```python
from build123d import *

# Parameters (mm, degrees)
SKETCH_R        = 1.6
PAD_DEPTH       = 9.5
SKETCH001_R     = 1.6
POCKET_DEPTH    = 8.001
POCKET_FACE6_W  = 8
POCKET_FACE6_H  = 9.5
PAD001_DEPTH    = 10
SKETCH002_R     = 1.6
POCKET001_DEPTH = 8.001


with BuildPart() as part:
    # Sketch → Pad (new body)
    with BuildSketch(Plane.XY):
        with BuildLine():
            ThreePointArc((0, -4), (4, 0), (0, 4))
            Line((0, 4), (-20, 4))
            Line((-20, 4), (-20, -4))
            Line((-20, -4), (0, -4))
        make_face()
        Circle(SKETCH_R, mode=Mode.SUBTRACT)
    extrude(amount=PAD_DEPTH)

    # Sketch001 (on Face2 of Pad) → Pocket (cut, through all)
    with BuildSketch(Plane(origin=(0, 4, 0), x_dir=(-1, 0, 0), z_dir=(0, 1, 0))):
        with Locations((15, 4.75)):
            Circle(SKETCH001_R)
    extrude(amount=-POCKET_DEPTH, mode=Mode.SUBTRACT)

    # Pocket Face6 → Pad001 (add)
    with BuildSketch(Plane(origin=(-20, 0, 4.75), x_dir=(0, 1, 0), z_dir=(-1, 0, 0))):
        Rectangle(POCKET_FACE6_W, POCKET_FACE6_H)
    extrude(amount=PAD001_DEPTH)

    # Sketch002 (on Face8 of Pad001) → Pocket001 (cut, through all)
    with BuildSketch(Plane(origin=(0, 4, 0), x_dir=(-1, 0, 0), z_dir=(0, 1, 0))):
        with Locations((25, 4.75)):
            Circle(SKETCH002_R)
    extrude(amount=-POCKET001_DEPTH, mode=Mode.SUBTRACT)


solid = part.part
```
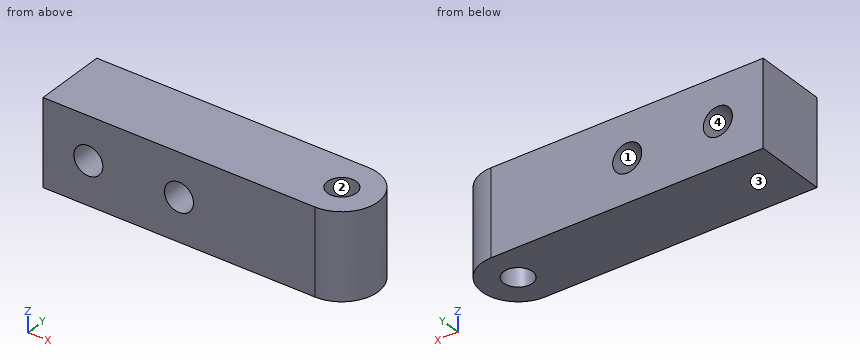
The listing builds one solid part. Answer for the finished solid, in the listing's coordinates (mm). Face numbers are marked on the shaded views. Coordinates: 2 decimals unless noted, no trailing zeros. Loops run counter-clockwise (first coordinate to the right, second up) from the corner with the lowest first, then second, coordinate; pieces in that order, holes last. Notation, with made-up numbers: (34.25, -40) - (85.25, -40) arc R11 ccw to (85.25, -23) - close; hole circle Ø6 at (88.25, 54). An arc over 180 degrees is marked (long way). Use a Markdown table: item, result. Add a question column.
1) The part is cut by section C-C, the plane x = -15. Give the vertices of the cut face in (y, z), and give its area (3 significant figures).
2) The part is cut by section B-B, the plane y = 0. Give the vertices of the cut face in (x, z), and give its area (3 significant figures).
3) The part is cut by section A-A, the plane z = 4.75. Give the vertices of the cut face in (x, y), and give its area (3 significant figures).
4) The part is cut by section D-D, the plane z = 1.75. Give the vertices of the cut face in (x, y), and give its area (3 significant figures).
5) Find the intervals of material crossed by line 1 (Z direction, x = -15, y = 0.75); line 2 (Y direction, x = -0.5, z = 7); line 3 (X direction, y = -1.25, z = 1), in increasing order.
6) The mould has two halves that part along Z. Classify the marked faces 1, 2, 3 and 4: released by +Z, released by -Z, zero draft, split by the parting line, or undercut.
Here are the results:
| question | item | result |
|---|---|---|
| 1 | outline | (-4, 0) - (4, 0) - (4, 3.15) - (-4, 3.15) - close; (-4, 6.35) - (4, 6.35) - (4, 9.5) - (-4, 9.5) - close |
| 1 | area | 50.4 mm^2 |
| 2 | outline | (-30, 0) - (-1.6, 0) - (-1.6, 9.5) - (-30, 9.5) - close; (1.6, 0) - (4, 0) - (4, 9.5) - (1.6, 9.5) - close; hole circle Ø3.2 at (-25, 4.75); hole circle Ø3.2 at (-15, 4.75) |
| 2 | area | 277 mm^2 |
| 3 | outline | (-30, -4) - (-26.6, -4) - (-26.6, 4) - (-30, 4) - close; (-23.4, -4) - (-16.6, -4) - (-16.6, 4) - (-23.4, 4) - close; (-13.4, -4) - (0, -4) arc R4 ccw to (0, 4) - (-13.4, 4) - close; hole circle Ø3.2 at (0, 0) |
| 3 | area | 206 mm^2 |
| 4 | outline | (-30, -4) - (0, -4) arc R4 ccw to (0, 4) - (-30, 4) - close; hole circle Ø3.2 at (0, 0) |
| 4 | area | 257 mm^2 |
| 5 | line 1 | z = 0 to 3.15, 6.35 to 9.5 |
| 5 | line 2 | y = -4 to -1.52, 1.52 to 4 |
| 5 | line 3 | x = -30 to -1, 1 to 3.8 |
| 6 | face 1 | undercut |
| 6 | face 2 | zero draft |
| 6 | face 3 | released by -Z |
| 6 | face 4 | undercut |
